```python
from build123d import *

# Parameters (mm, degrees)
BOSS_EXTRUDE2_DEPTH = 10
SKETCH2_R           = 1.6
CUT_EXTRUDE1_DEPTH  = 10
SKETCH3_R           = 1.6
CUT_EXTRUDE2_DEPTH  = 10


with BuildPart() as part:
    # Sketch1 → Boss-Extrude2 (new body)
    with BuildSketch(Plane(origin=(0, 0, 0), x_dir=(1, 0, 0), z_dir=(0, 1, 0))):
        Polygon((0, 0), (0, 20), (3, 20), (3, 3), (25, 3), (25, 0), align=None)
    extrude(amount=BOSS_EXTRUDE2_DEPTH)

    # Sketch2 → Cut-Extrude1 (cut)
    with BuildSketch(Plane.XY):
        with Locations((20, 5)):
            Circle(SKETCH2_R)
        with Locations((10, 5)):
            Circle(SKETCH2_R)
    extrude(amount=-CUT_EXTRUDE1_DEPTH, mode=Mode.SUBTRACT)

    # Sketch3 → Cut-Extrude2 (cut)
    with BuildSketch(Plane(origin=(3, 0, 0), x_dir=(0, 0, -1), z_dir=(1, 0, 0))):
        with Locations((7.5, 5)):
            Circle(SKETCH3_R)
        with Locations((17.5, 5)):
            Circle(SKETCH3_R)
    extrude(amount=-CUT_EXTRUDE2_DEPTH, mode=Mode.SUBTRACT)


solid = part.part
```
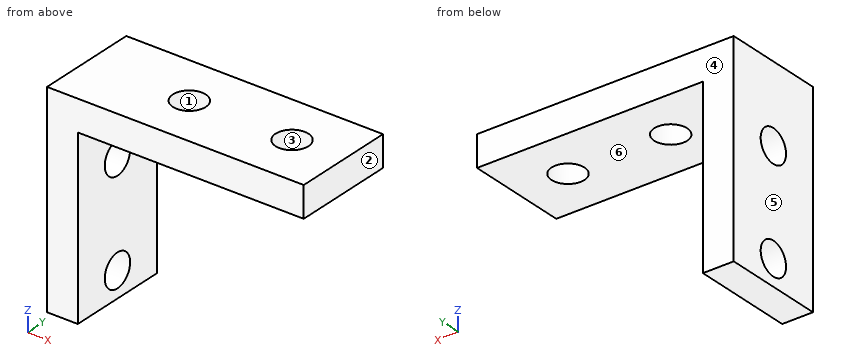
Verification items for the finished model (mm, model axes). Face numbers are marked on the shaded views. A direction names the side the tool comes from. Coordinates: 2 decimals unless noted, no trailing zeros. Write each loop counter-clockwise with the first axis right and the second up, starting at its lowest first coordinate (ties: lowest second). Pieces come first, ordered by that corner, then holes. Notation, with made-up numbers: M 38,-0.5 L 93,-0.5 A30 ccw 93,26.5 Z; hole C 54.5,-17.5 d11. An arc over 180 degrees is marked long. One line per item, written item: value.
Item 1: Section check A-A, the plane z = -7.5. Record the boundary of the cut face in (x, y), plus the area to 3 significant figures.
Check sheet entries:
outline: M 0,0 L 3,0 L 3,3.4 L 0,3.4 Z; M 0,6.6 L 3,6.6 L 3,10 L 0,10 Z
area: 20.4 mm^2
Item 2: Section check C-C, the plane x = 20. Record the boundary of the cut face in (y, z).
Check sheet entries:
outline: M 0,-3 L 3.4,-3 L 3.4,0 L 0,0 Z; M 6.6,-3 L 10,-3 L 10,0 L 6.6,0 Z
Item 3: Gauge pin test, flat ends, axial feed: pin 1 Ø3 at (x, y) = (7.5, 2) entering from -Z; pin 2 Ø1 at (y, z) = (6.5, -11.5) entering from +X. Record the tip position at first contact, or that the pin passes through.
Check sheet entries:
pin 1: stops at z = -3
pin 2: stops at x = 3
Item 4: Section check D-D, the plane y = 7.75. Record the boundary of the cut face in (x, z).
Check sheet entries:
outline: M 0,-20 L 3,-20 L 3,-3 L 25,-3 L 25,0 L 0,0 Z
Item 5: Mould release check, pull along X, two halves, no side actions. Record for the marked faces 1, 2, 3 and 4: pulls with the +X half, pulls with the -X half, needs draft (parallel to the pull), parting line crosses it, or undercut.
Check sheet entries:
face 1: undercut
face 2: pulls with the +X half
face 3: undercut
face 4: needs draft
Item 6: Section check B-B, the plane y = 5. Record the boundary of the cut face in (x, z), plus the area to 3 significant figures.
Check sheet entries:
outline: M 0,-20 L 3,-20 L 3,-19.1 L 0,-19.1 Z; M 0,-15.9 L 3,-15.9 L 3,-9.1 L 0,-9.1 Z; M 0,-5.9 L 3,-5.9 L 3,-3 L 8.4,-3 L 8.4,0 L 0,0 Z; M 11.6,-3 L 18.4,-3 L 18.4,0 L 11.6,0 Z; M 21.6,-3 L 25,-3 L 25,0 L 21.6,0 Z
area: 87.6 mm^2
Item 7: Access from +Z, -Z, +X, -X, +Y, -Y to the whole of each face (thin tool, end or side, straight path). Record for the marked faces 5 and 6.
Check sheet entries:
face 5: +Z, -Z, -X, +Y, -Y
face 6: -Z, +X, +Y, -Y
Item 8: Scan lines: line 1 along Y through (x, z) = (1.25, -17.5); line 2 along Z through (x, y) = (14.5, 6.5); line 3 along X through (y, z) = (8, -7). Record each from-to range of solid material in increasing order.
Check sheet entries:
line 1: y = 0 to 3.4, 6.6 to 10
line 2: z = -3 to 0
line 3: x = 0 to 3
